The model under review builds one solid part; all positions refer to its coordinate system, in mm. Face numbers are marked on the shaded views. A direction names the side the tool comes from. Coordinates: 2 decimals unless noted, no trailing zeros. Write each loop counter-clockwise with the first axis right and the second up, starting at its lowest first coordinate (ties: lowest second). Pieces come first, ordered by that corner, then holes.
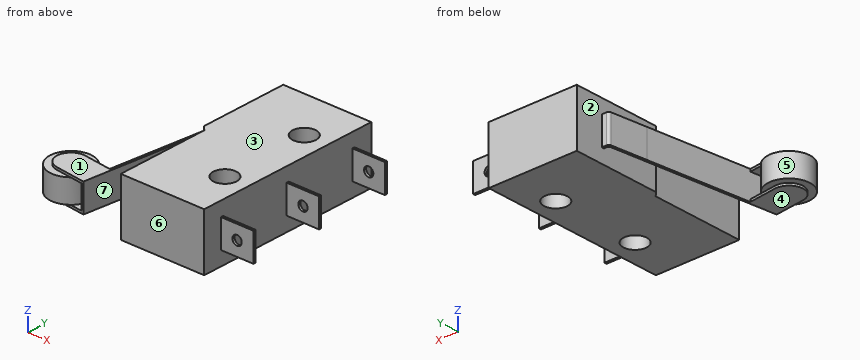
```python
from build123d import *

# Parameters (mm, degrees)
SKETCH_1_R           = 1.25
EXTRUDE_1_DEPTH      = 6
EXTRUDE_2_DEPTH      = 1.5
EXTRUDE_2_DEPTH_BACK = 1.5
EXTRUDE_3_DEPTH      = 0.25
SKETCH_5_R           = 2.25
EXTRUDE_4_DEPTH      = 2.5
SKETCH_6_W           = 3
SKETCH_6_H           = 0.25
EXTRUDE_5_DEPTH      = 3.5
SKETCH_7_R           = 0.5
CUT_EXTRUDE_1_DEPTH  = 20.250480762


with BuildPart() as part:
    # Эскиз1 → Бобышка-Вытянуть1 (new body)
    with BuildSketch(Plane.XY):
        Polygon((0, 0), (0, 10), (-0.5, 10.5), (-0.5, 20), (0, 20), (9, 20), (9, 0), align=None)
        with Locations((6.5, 5.25)):
            Circle(SKETCH_1_R, mode=Mode.SUBTRACT)
        with Locations((6.5, 14.75)):
            Circle(SKETCH_1_R, mode=Mode.SUBTRACT)
    extrude(amount=EXTRUDE_1_DEPTH)

    # Эскиз3 → Бобышка-Вытянуть2 (add, two sides)
    with BuildSketch(Plane(origin=(0, 0, 3), x_dir=(0, -1, 0), z_dir=(0, 0, -1))) as extrude_2_sk:
        with BuildLine():
            Line((-17, 0.5), (-17, 1.029304445))
            ThreePointArc((-17, 1.029304445), (-16.937419544, 1.194755086), (-16.781008684, 1.277373915))
            Line((-16.781008684, 1.277373915), (-13, 1.75))
            Line((-13, 1.75), (0.861001781, 3.482625223))
            Line((0.861001781, 3.482625223), (0.892010464, 3.234555753))
            Line((0.892010464, 3.234555753), (-16.531008684, 1.05667836))
            ThreePointArc((-16.531008684, 1.05667836), (-16.687419544, 0.974059532), (-16.75, 0.808608891))
            Line((-16.75, 0.808608891), (-16.75, 0.5))
            Line((-16.75, 0.5), (-17, 0.5))
        make_face()
    extrude(amount=EXTRUDE_2_DEPTH)
    extrude(extrude_2_sk.sketch, amount=-EXTRUDE_2_DEPTH_BACK)

    # Эскиз4 → Бобышка-Вытянуть3 (add)
    with BuildSketch(Plane.XY.offset(4.5)):
        with BuildLine():
            Line((-3.482625223, -0.861001781), (-6.459458853, -0.488897577))
            ThreePointArc((-6.459458853, -0.488897577), (-7.761823566, 1.18557134), (-6.087354649, 2.487936053))
            Line((-6.087354649, 2.487936053), (-3.110521019, 2.115831849))
            Line((-3.110521019, 2.115831849), (-3.482625223, -0.861001781))
        make_face()
    extrude_3 = extrude(amount=-EXTRUDE_3_DEPTH)

    # Зеркальное отражение1: Бобышка-Вытянуть3 across plane
    add(extrude_3.mirror(Plane(origin=(0, 0, 3), x_dir=(1, 0, 0), z_dir=(0, 0, -1))))

    # Эскиз5 → Бобышка-Вытянуть4 (add)
    with BuildSketch(Plane(origin=(0, 0, 4.25), x_dir=(-1, 0, 0), z_dir=(0, 0, -1))):
        with Locations((6.273406751, 0.999519238)):
            Circle(SKETCH_5_R)
    extrude(amount=EXTRUDE_4_DEPTH)

    # Эскиз6 → Бобышка-Вытянуть5 (add)
    with BuildSketch(Plane(origin=(9, 0, 0), x_dir=(0, 0, -1), z_dir=(1, 0, 0))):
        with Locations((-3, 2.125)):
            Rectangle(SKETCH_6_W, SKETCH_6_H)
        with Locations((-3, 17.875)):
            Rectangle(SKETCH_6_W, SKETCH_6_H)
        with Locations((-3, 10)):
            Rectangle(SKETCH_6_W, SKETCH_6_H)
    extrude(amount=EXTRUDE_5_DEPTH)

    # Эскиз7 → Вырез-Вытянуть1 (cut, through all)
    with BuildSketch(Plane(origin=(0, 18, 0), x_dir=(1, 0, 0), z_dir=(0, 1, 0))):
        with Locations((10.75, -3)):
            Circle(SKETCH_7_R)
    extrude(amount=-CUT_EXTRUDE_1_DEPTH, mode=Mode.SUBTRACT)


solid = part.part
```
Item 1: To check wall thickness, follow line 1 along Y through (x, z) = (6.5, 4.75); line 2 along X through (y, z) = (17.9, 3); line 3 along Z through (x, y) = (10.75, 10). State the ranges of each line that lie inside material, in increasing order.
Solved:
line 1: y = 0 to 4, 6.5 to 13.5, 16 to 20
line 2: x = -0.5 to 10.25, 11.25 to 12.5
line 3: z = 1.5 to 2.5, 3.5 to 4.5
Item 2: Take a section at A-A, the plane x = 6.5. Write out the cut boundary in (y, z).
Solved:
outline: (0, 0) - (4, 0) - (4, 6) - (0, 6) - close; (6.5, 0) - (13.5, 0) - (13.5, 6) - (6.5, 6) - close; (16, 0) - (20, 0) - (20, 6) - (16, 6) - close
Item 3: For pin 1 (3.5 mm diameter, centred on x = 11.5, z = 3.5, fed in from +Y); pin 2 (1.8 mm diameter, centred on y = 13.5, z = 3, fed in from -X); pin 3 (0.9 mm diameter, centred on x = 11.5, z = 2.5, fed in from -Y), all flat-tipped, find the tip position at first contact; note any pin that passes through.
Solved:
pin 1: stops at y = 18
pin 2: stops at x = -1.8
pin 3: stops at y = 2
Item 4: Mouldability with a two-part tool opening along X and no side actions: class the marked faces 1 and 2 as pulls with the +X half, pulls with the -X half, needs draft (parallel to the pull), parting line crosses it, or undercut.
Solved:
face 1: needs draft
face 2: undercut
Item 5: Take a section at C-C, the plane z = 0.85. Write out the cut boundary in (x, y), plus the area to 3 significant figures.
Solved:
outline: (-0.5, 10.5) - (0, 10) - (0, 0) - (9, 0) - (9, 20) - (-0.5, 20) - close; hole circle Ø2.5 at (6.5, 5.25); hole circle Ø2.5 at (6.5, 14.75)
area: 175 mm2
Item 6: Machinability: for the marked faces 3, 4, 5, 6 and 7, which of the approach directions +Z, -Z, +X, -X, +Y, -Y give a long, thin tool a straight path to every point of the face, cutting with its end or side? Answer none if there is none.
Solved:
face 3: +Z, +X, -X, +Y, -Y
face 4: -Z, -X, +Y, -Y
face 5: none
face 6: +Z, -Z, +X, -Y
face 7: +Z, -Z, -Y
Item 7: Take a section at B-B, the plane x = 10.75. Write out the cut boundary in (y, z) (3 decimals).
Solved:
outline: (2, 1.5) - (2.25, 1.5) - (2.25, 2.5) - (2, 2.5) - close; (2, 3.5) - (2.25, 3.5) - (2.25, 4.5) - (2, 4.5) - close; (9.875, 1.5) - (10.125, 1.5) - (10.125, 2.5) - (9.875, 2.5) - close; (9.875, 3.5) - (10.125, 3.5) - (10.125, 4.5) - (9.875, 4.5) - close; (17.75, 1.5) - (18, 1.5) - (18, 2.5) - (17.75, 2.5) - close; (17.75, 3.5) - (18, 3.5) - (18, 4.5) - (17.75, 4.5) - close
Item 8: Take a section at D-D, the plane y = 16.25. Write out the cut boundary in (x, z).
Solved:
outline: (-1.34, 1.5) - (-1.09, 1.5) - (-1.09, 4.5) - (-1.34, 4.5) - close; (-0.5, 0) - (9, 0) - (9, 6) - (-0.5, 6) - close
